Answer from the drawing. Dimensions are ordinates in mm from the lowest x, y and z of the part. Coordinates: 2 decimals unless noted, no trailing zeros. Loops run counter-clockwise (first coordinate to the right, second up) from the corner with the lowest first, then second, coordinate; pieces in that order, holes last.
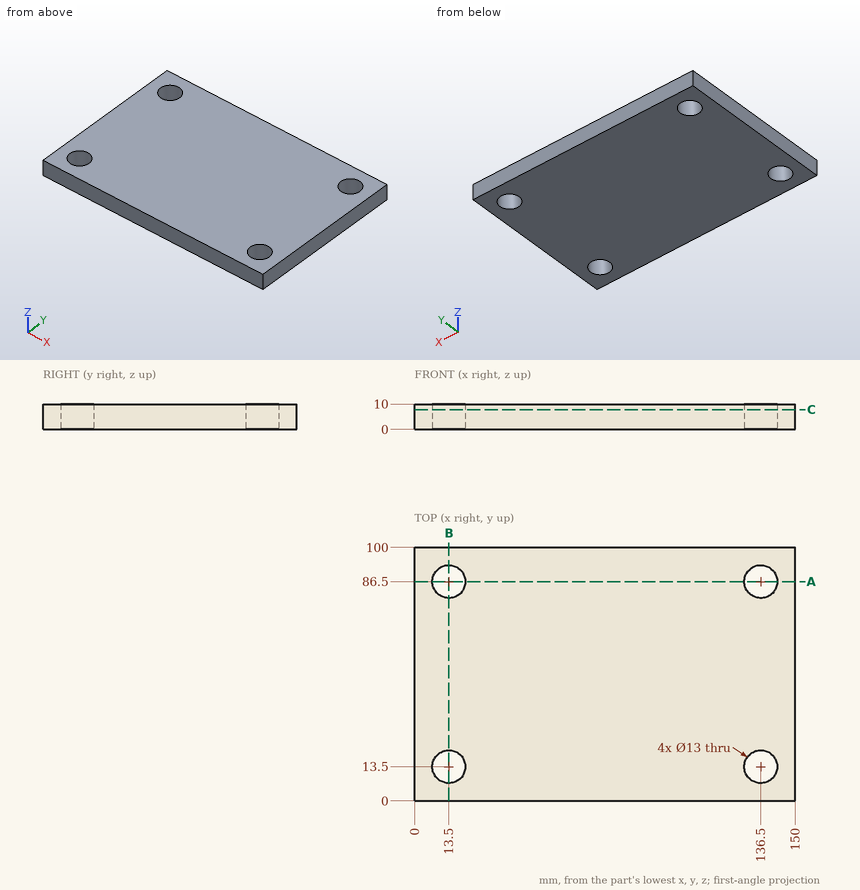
Item 1: A cutting plane is placed at C-C on z = 7.75. Determine the outline of the cut face in (x, y).
Numbers:
outline: (0, 0) - (150, 0) - (150, 100) - (0, 100) - close; hole circle Ø13 at (13.5, 13.5); hole circle Ø13 at (13.5, 86.5); hole circle Ø13 at (136.5, 13.5); hole circle Ø13 at (136.5, 86.5)
Item 2: A cutting plane is placed at A-A on y = 86.5. Determine the outline of the cut face in (x, z), then the cut area to 3 significant figures.
Numbers:
outline: (0, 0) - (7, 0) - (7, 10) - (0, 10) - close; (20, 0) - (130, 0) - (130, 10) - (20, 10) - close; (143, 0) - (150, 0) - (150, 10) - (143, 10) - close
area: 1,240 mm2
Item 3: Find the intervals of material crossed by line 1 along Y through (x, z) = (13.5, 4); line 2 along X through (y, z) = (81, 3.75); line 3 along Y through (x, z) = (138.5, 7), in increasing order.
Numbers:
line 1: y = 0 to 7, 20 to 80, 93 to 100
line 2: x = 0 to 10.04, 16.96 to 133.04, 139.96 to 150
line 3: y = 0 to 7.32, 19.68 to 80.32, 92.68 to 100
Item 4: A cutting plane is placed at B-B on x = 13.5. Determine the outline of the cut face in (y, z), then the cut area to 3 significant figures.
Numbers:
outline: (0, 0) - (7, 0) - (7, 10) - (0, 10) - close; (20, 0) - (80, 0) - (80, 10) - (20, 10) - close; (93, 0) - (100, 0) - (100, 10) - (93, 10) - close
area: 740 mm2
Item 5: Given pin 1 (1.5 mm diameter, centred on x = 44, y = 67.5, fed in from -Z); pin 2 (8 mm diameter, centred on x = 13.5, y = 86.5, fed in from -Z), each flat-ended and moving along its own axis, determine where each tip first touches the part or whether it passes through.
Numbers:
pin 1: stops at z = 0
pin 2: passes through
